from build123d import *
from OCP.BRepFilletAPI import BRepFilletAPI_MakeChamfer

# Parameters (mm, degrees)
SKETCH1_R               = 4.765
BOSS_EXTRUDE1_DEPTH     = 9.5
CHAMFER5_SIZE           = 7.62
CHAMFER5_SIZE2          = 2.54
CHAMFER6_SIZE           = 2.54
CHAMFER6_SIZE2          = 7.62
SKETCH2_W               = 9.53
SKETCH2_H               = 9.53
CUT_EXTRUDE1_DEPTH      = 32.662585176
SKETCH2_2_W             = 9.53
SKETCH2_2_H             = 9.53
CUT_EXTRUDE2_DEPTH      = 32.662585176
CUT_EXTRUDE3_DEPTH      = 32.662585176
CUT_EXTRUDE3_DEPTH_BACK = 32.662585176
CUT_EXTRUDE4_DEPTH      = 32.662585236
CUT_EXTRUDE4_DEPTH_BACK = 32.662585236
SKETCH4_R               = 1.59


with BuildPart() as part:
    # Sketch1 → Boss-Extrude1 (new, symmetric)
    with BuildSketch(Plane.XY):
        with BuildLine():
            Line((0, 9.77), (-22.23, 9.77))
            Line((-22.23, 9.77), (-22.23, 4.77))
            Line((-22.23, 4.77), (-9.711509246, -1.067468107))
            ThreePointArc((-9.711509246, -1.067468107), (-5.694059685, -7.939180329), (2.103028838, -9.540973206))
            Line((2.103028838, -9.540973206), (28.58, -5))
            Line((28.58, -5), (28.58, 0))
            Line((28.58, 0), (9.77, 0))
            ThreePointArc((9.77, 0), (6.908433252, 6.908433252), (0, 9.77))
        make_face()
        Circle(SKETCH1_R, mode=Mode.SUBTRACT)
    extrude(amount=BOSS_EXTRUDE1_DEPTH, both=True)

    # Chamfer5
    chamfer5_edges = [part.edges().sort_by_distance(p)[0] for p in [
        (-22.23, 7.27, -9.5),
        (28.58, -2.5, -9.5),
    ]]
    chamfer5_side = [part.faces().sort_by_distance(p)[0] for p in [
        (6.52350029, 6.52350029, -9.5),
    ]]
    chamfer(chamfer5_edges, length=CHAMFER5_SIZE, length2=CHAMFER5_SIZE2, reference=chamfer5_side[0])

    # Chamfer6: one chamfer whose edges measure the first distance from different faces: ONE call of the kernel's chamfer builder (chamfer() names one face for all edges)
    chamfer6_edges_1 = [part.edges().sort_by_distance(p)[0] for p in [
        (-22.23, 7.27, 9.5),
    ]]
    chamfer6_side_1 = [part.faces().sort_by_distance(p)[0] for p in [
        (-22.23, 7.27, 1.27),
    ]]
    chamfer6_edges_2 = [part.edges().sort_by_distance(p)[0] for p in [
        (28.58, -2.5, 9.5),
    ]]
    chamfer6_side_2 = [part.faces().sort_by_distance(p)[0] for p in [
        (28.58, -2.5, 1.27),
    ]]
    chamfer6 = BRepFilletAPI_MakeChamfer(part.part.solid().wrapped)
    for e in chamfer6_edges_1:
        chamfer6.Add(CHAMFER6_SIZE, CHAMFER6_SIZE2, e.wrapped, chamfer6_side_1[0].wrapped)  # the first distance lies on this face
    for e in chamfer6_edges_2:
        chamfer6.Add(CHAMFER6_SIZE, CHAMFER6_SIZE2, e.wrapped, chamfer6_side_2[0].wrapped)  # the first distance lies on this face
    add(Compound.cast(chamfer6.Shape()), mode=Mode.REPLACE)

    # Sketch2 → Cut-Extrude1 (cut, through all)
    with BuildSketch(Plane(origin=(0, 0, 0), x_dir=(1, 0, 0), z_dir=(0, 1, 0))):
        with Locations((-17.465, 0)):
            Rectangle(SKETCH2_W, SKETCH2_H)
        with Locations((23.815, 0)):
            Rectangle(SKETCH2_W, SKETCH2_H)
    extrude(amount=-CUT_EXTRUDE1_DEPTH, mode=Mode.SUBTRACT)

    # Sketch2<2> → Cut-Extrude2 (cut, through all)
    with BuildSketch(Plane(origin=(0, 0, 0), x_dir=(1, 0, 0), z_dir=(0, 1, 0))):
        with Locations((-17.465, 0)):
            Rectangle(SKETCH2_2_W, SKETCH2_2_H)
        with Locations((23.815, 0)):
            Rectangle(SKETCH2_2_W, SKETCH2_2_H)
    extrude(amount=CUT_EXTRUDE2_DEPTH, mode=Mode.SUBTRACT)

    # Sketch3 → Cut-Extrude3 (cut, two sides: drawn at the far end of the back side and taken through both)
    with BuildSketch(Plane(origin=(0, 0, 0), x_dir=(1, 0, 0), z_dir=(0, 1, 0)).offset(-CUT_EXTRUDE3_DEPTH_BACK)):
        with BuildLine():
            Line((-3.81, 5.08), (6.35, 5.08))
            ThreePointArc((6.35, 5.08), (11.43, 0), (6.35, -5.08))
            Line((6.35, -5.08), (-3.81, -5.08))
            ThreePointArc((-3.81, -5.08), (-8.89, 0), (-3.81, 5.08))
        make_face()
    extrude(amount=CUT_EXTRUDE3_DEPTH + CUT_EXTRUDE3_DEPTH_BACK, mode=Mode.SUBTRACT)

    # Sketch4 → Cut-Extrude4 (cut, two sides: drawn at the far end of the back side and taken through both)
    with BuildSketch(Plane.XY.offset(-CUT_EXTRUDE4_DEPTH_BACK)):
        with Locations((-19.69, 7.23)):
            Circle(SKETCH4_R)
        with Locations((26.04, -2.54)):
            Circle(SKETCH4_R)
    extrude(amount=CUT_EXTRUDE4_DEPTH + CUT_EXTRUDE4_DEPTH_BACK, mode=Mode.SUBTRACT)


solid = part.part
Can you work these out from the model? Positions are in its coordinate system, mm. A direction names the side the tool comes from. Round coordinates to 2 decimals unless told otherwise and drop trailing zeros. Write each loop counter-clockwise with the first axis right and the second up, starting at its lowest first coordinate (ties: lowest second). Pieces come first, ordered by that corner, then holes. Notation, with made-up numbers: M 69,38.5 L 107,38.5 A20 cw 107,77.5 Z; hole C 46,63 d6. An arc over 180 degrees is marked long. Use a Markdown table: item, result.
Item 1: I want a section at C-C (x = 12). List the corners of the cut face in (y, z) for me.
Found:
| item | result |
|---|---|
| outline | M -7.84,-9.5 L 0,-9.5 L 0,9.5 L -7.84,9.5 Z |
Item 2: For pin 1 Ø2 at (x, y) = (24.5, -3.5) entering from -Z; pin 2 Ø8 at (x, z) = (6, 3) entering from -Y; pin 3 Ø8 at (y, z) = (-7.5, 3) entering from -X; pin 4 Ø1.9 at (x, y) = (-19.69, 7.23) entering from +Z, each with a flat end and sliding along its axis, tell me the tip position at first contact or that it passes through.
Found:
| item | result |
|---|---|
| pin 1 | stops at z = -8.65 |
| pin 2 | stops at y = -9.46 |
| pin 3 | stops at x = -9.12 |
| pin 4 | passes through |
Item 3: I want a section at B-B (x = -19.69). List the corners of the cut face in (y, z) for me (3 decimals).
Found:
| item | result |
|---|---|
| outline | M 3.586,-7.807 L 5.64,-7.807 L 5.64,-4.765 L 3.586,-4.765 Z; M 3.586,4.765 L 5.64,4.765 L 5.64,7.807 L 3.586,7.807 Z; M 8.82,-7.807 L 9.77,-7.807 L 9.77,-4.765 L 8.82,-4.765 Z; M 8.82,4.765 L 9.77,4.765 L 9.77,7.807 L 8.82,7.807 Z |
Item 4: I want a section at A-A (z = 0). List the corners of the cut face in (x, y) for me.
Found:
| item | result |
|---|---|
| outline | M -12.7,0.33 L -9.71,-1.07 A9.77 ccw -8.89,-4.05 L -8.89,9.77 L -12.7,9.77 Z; M 11.43,-7.94 L 19.05,-6.63 L 19.05,0 L 11.43,0 Z |
Item 5: Which directions (+Z, -Z, +X, -X, +Y, -Y) give clear straight access to the entire face, cutting with the end or side of a thin tool? Please do faces 4 (the face through (-22.23, 7, 6)), 5 (the face through (23, -3, -4.765)), 6 (the face through (-16, 6, -4.765)).
Found:
| item | result |
|---|---|
| face 4 | +Z, -Z, -X, +Y, -Y |
| face 5 | +X, +Y, -Y |
| face 6 | -X, +Y, -Y |
Item 6: We'd pull the mould along Y, two halves only. Please class faces 1 (the face through (5, -2, -5.08)), 2 (the face through (17, 0, 0)), 3 (the face through (-0.62, 4.724, 7.213)): released by +Y, released by -Y, zero draft, split by the parting line, or undercut.
Found:
| item | result |
|---|---|
| face 1 | zero draft |
| face 2 | released by +Y |
| face 3 | undercut |
Item 7: If I drill on line 1 along Z through (x, y) = (0.5, -7.25); line 2 along X through (y, z) = (-2.54, 5.55); line 3 along X through (y, z) = (-2, 4.5), over which ranges is the centre line in solid material (lowest first)? Write a range as [from, to].
Found:
| item | result |
|---|---|
| line 1 | z = [-9.5, -5.08], [5.08, 9.5] |
| line 2 | x = [-9.43, -4.03], [4.03, 24.45], [27.63, 28.58] |
| line 3 | x = [-9.56, -6.17], [8.71, 19.05] |
Item 8: I want a section at D-D (z = 2.5). List the corners of the cut face in (x, y) for me, and give its area (3 significant figures).
Found:
| item | result |
|---|---|
| outline | M -12.7,0.33 L -9.71,-1.07 A9.77 ccw -8.23,-5.26 L -8.23,9.77 L -12.7,9.77 Z; M 10.77,-8.05 L 19.05,-6.63 L 19.05,0 L 10.77,0 Z |
| area | 111 mm2 |
